Verification items for this drawing (mm, ordinates from the low corner). Coordinates: 2 decimals unless noted, no trailing zeros. Loops run counter-clockwise (first coordinate to the right, second up) from the corner with the lowest first, then second, coordinate; pieces in that order, holes last. Notation, with made-up numbers: (-27.75, 30.5) - (2.25, 30.5) arc R20 cw to (2.25, 51.5) - close; hole circle Ø2 at (54.5, 50.25). An arc over 180 degrees is marked (long way). One line per item, written item: value. Start each with the question number.
(1) Section check D-D (x = 13.5). Record the boundary of the cut face in (y, z).
(2) Gauge pin test, flat end, axial feed: P1, Ø5.5, axis at x = 42, z = 6, coming from the +Y side. Record the tip position at first contact, or that the pin passes through.
(3) Section check C-C (x = 41). Record the boundary of the cut face in (y, z), plus the area to 3 significant figures.
(4) Section check A-A (y = 5.25). Record the boundary of the cut face in (x, z), plus the area to 3 significant figures.
(5) Draft check along X on the marked faces 1, 2, 3 and 4. Enter one of: +X half, -X half, draft (parallel to the pull), parting line (faces both ways), or undercut.
(6) Thickness scan on probe 1 along Z at (x, y) = (16, 2.75); probe 2 along X at (y, z) = (9, 5); probe 3 along X at (y, z) = (10.5, 3.5). Record the ranges inside material, lowest first. Write a range as [from, to].
(7) Section check B-B (z = 6). Record the boundary of the cut face in (x, y).
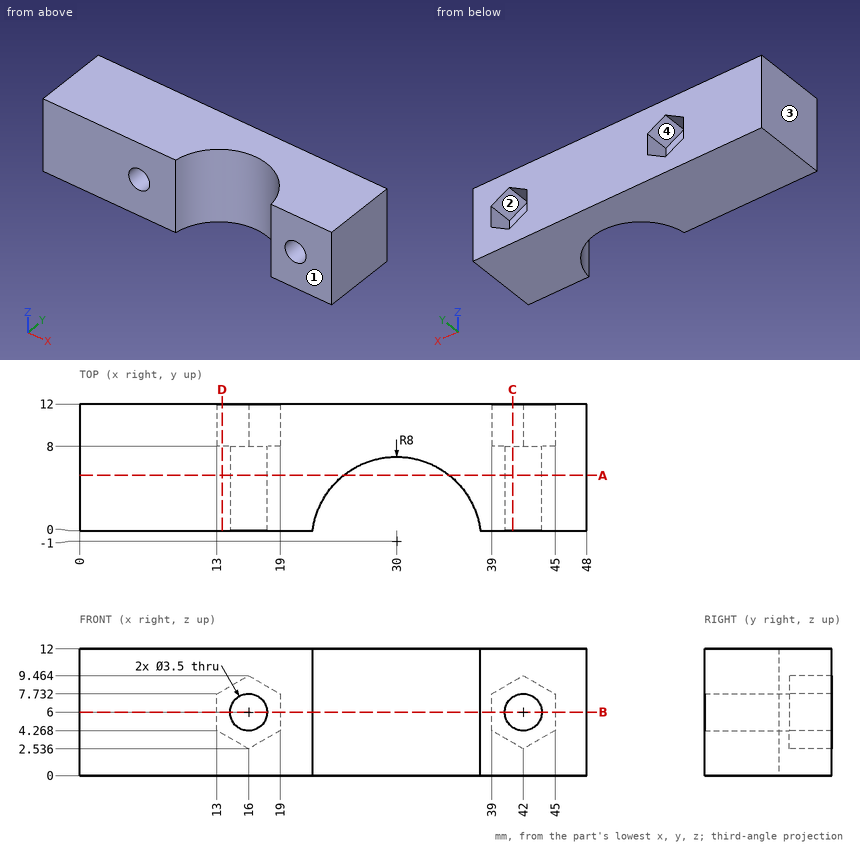
Responses:
1. outline: (0, 0) - (12, 0) - (12, 3.98) - (8, 3.98) - (8, 8.02) - (12, 8.02) - (12, 12) - (0, 12) - close
2. P1: stops at y = 8
3. outline: (0, 0) - (12, 0) - (12, 3.11) - (8, 3.11) - (8, 4.56) - (0, 4.56) - close; (0, 7.44) - (8, 7.44) - (8, 8.89) - (12, 8.89) - (12, 12) - (0, 12) - close
3. area: 97.9 mm²
4. outline: (0, 0) - (25.01, 0) - (25.01, 12) - (0, 12) - close; (34.99, 0) - (48, 0) - (48, 12) - (34.99, 12) - close; hole circle Ø3.5 at (16, 6); hole circle Ø3.5 at (42, 6)
4. area: 437 mm²
5. face 1: draft
5. face 2: undercut
5. face 3: -X half
5. face 4: undercut
6. probe 1: z = [0, 4.25], [7.75, 12]
6. probe 2: x = [0, 13], [19, 39], [45, 48]
6. probe 3: x = [0, 14.33], [17.67, 40.33], [43.67, 48]
7. outline: (0, 0) - (14.25, 0) - (14.25, 8) - (13, 8) - (13, 12) - (0, 12) - close; (17.75, 0) - (22.06, 0) arc R8 cw to (37.94, 0) - (40.25, 0) - (40.25, 8) - (39, 8) - (39, 12) - (19, 12) - (19, 8) - (17.75, 8) - close; (43.75, 0) - (48, 0) - (48, 12) - (45, 12) - (45, 8) - (43.75, 8) - close
